```python
from build123d import *

# Parameters (mm, degrees)
F1_DEPTH = 40
F3_DEPTH = 12.5
F4_R     = 2.2
F5_DEPTH = 12.501
F7_SIZE  = 2
F6_R     = 4.65
F8_DEPTH = 1
F9_SIZE  = 2.44999


# Not quite as in the source:
# - a fillet or chamfer is up to 0.001 mm smaller than in the source, because OpenCascade refuses the exact size


with BuildPart() as f1:
    # F0 (on Top) → F1 (new body)
    with BuildSketch(Plane.XY):
        Polygon((2, 10), (-10.5, 10), (-10.5, 0), (0, 0), (0, -7.5), (1, -7.5), (5.5, -1), (2, -1), align=None)
    extrude(amount=F1_DEPTH)

    # F2 (on face) → F3 (cut, symmetric)
    with BuildSketch(Plane.XZ):
        with BuildLine():
            ThreePointArc((-2, 35.8), (-1, 34.8), (0, 35.8))
            Line((0, 35.8), (5.5, 35.8))
            Line((5.5, 35.8), (5.5, 40))
            Line((5.5, 40), (-10.5, 40))
            Line((-10.5, 40), (-10.5, 33.8))
            Line((-10.5, 33.8), (-3, 35.8))
            Line((-3, 35.8), (-2, 35.8))
        make_face()
    extrude(amount=F3_DEPTH, both=True, mode=Mode.SUBTRACT)

    # F4 (on face) → F5 (cut, through all)
    with BuildSketch(Plane.YZ.offset(2)):
        with Locations((4.5, 25.8)):
            Circle(F4_R)
        with Locations((4.5, 10)):
            Circle(F4_R)
    extrude(amount=-F5_DEPTH, mode=Mode.SUBTRACT)

    # F7
    f7_edges = [f1.edges().sort_by_distance(p)[0] for p in [
        (-10.5, 10, 16.9),
    ]]
    chamfer(f7_edges, length=F7_SIZE)

    # F6 (on face) → F8 (cut)
    with BuildSketch(Plane.YZ.offset(2)):
        with Locations((4.5, 25.8)):
            Circle(F6_R)
        with Locations((4.5, 10)):
            Circle(F6_R)
    extrude(amount=-F8_DEPTH, mode=Mode.SUBTRACT)

    # F9 (size 2.45 in the source; OpenCascade refuses exactly that, so slightly less here)
    f9_edges = [f1.edges().sort_by_distance(p)[0] for p in [
        (1, 2.3, 25.8),
        (1, 2.3, 10),
    ]]
    chamfer(f9_edges, length=F9_SIZE)


solid = f1.part
```
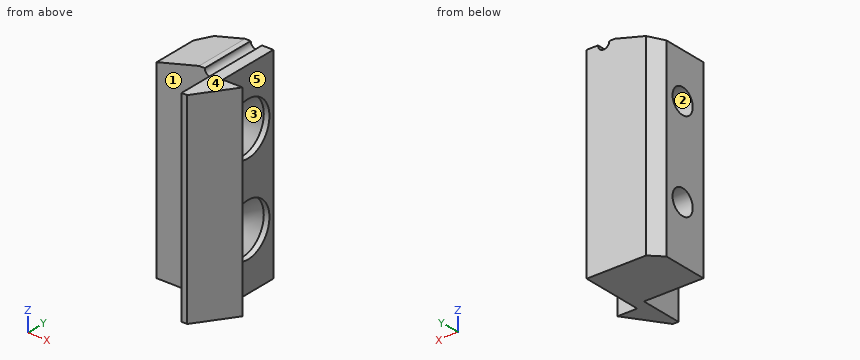
Read the model definition and answer for the solid it produces. Units are mm, in the model's axes. Face numbers are marked on the shaded views. A direction names the side the tool comes from. Coordinates: 2 decimals unless noted, no trailing zeros. Order: outer loops, then holes, each group sorted by start corner. A loop starts at its lowest first (then second) coordinate and runs counter-clockwise, first axis right, second up. Notation, with made-up numbers: (25.5, -27) - (71.5, -27) arc R26 ccw to (71.5, 5) - close; hole circle Ø8 at (30, 61.25). An arc over 180 degrees is marked (long way). Answer as a JSON object with one key per item and string values. Group by question number.
Item 1: Section D-D (z = 31.5) is taken. Give the vertices of the cut face in (x, y), plus the area to 3 significant figures.
Item 2: The mould has two halves that part along Z. Classify the marked faces 3, 4 and 5: +Z half, -Z half, draft (parallel to the pull), parting line (faces both ways), or undercut.
Item 3: Consider probe 1 along Z at (x, y) = (1.3, 4.5); probe 2 along Z at (x, y) = (-3.75, 4.5); probe 3 along X at (y, z) = (2.25, 20). Determine where each line is inside the solid, lowest interval first. Write a range as from..to.
Item 4: Section B-B (y = 4.5) is taken. State how many separate pieces and enclosed holes the cut face has, plus the area to 3 significant figures.
Item 5: Section C-C (x = -6) is taken. Give the vertices of the cut face in (y, z).
Item 6: A tool of negligible diameter and unlimited length cuts with its end or side. For the marked faces 1 and 2, from which of +Z, -Z, +X, -X, +Y, -Y can it reach the whole face along a straight path? Write none if from no direction.
Item 7: Flat-ended cylindrical pins translate along their axes: P1, Ø5, axis at x = -4.5, z = 17.5, coming from the -Y side; P2, Ø1, axis at x = 4.5, z = 17, coming from the +Y side; P3, Ø6, axis at y = 3.5, z = 27.5, coming from the +X side. Find the tip coordinate at first contact, or state that the pin passes through.
Results are:
{
 "1": {"outline": "(-10.5, 0) - (0, 0) - (0, -7.5) - (1, -7.5) - (5.5, -1) - (2, -1) - (2, 10) - (-8.5, 10) - (-10.5, 8) - close", "area": "146 mm^2"},
 "2": {"face 3": "undercut", "face 4": "+Z half", "face 5": "draft"},
 "3": {"probe 1": "z = 0..5.35, 14.65..21.15, 30.45..35.8", "probe 2": "z = 0..7.8, 12.2..23.6, 28..35.6", "probe 3": "x = -10.5..2"},
 "4": {"separate pieces": "3", "enclosed holes": "0", "area": "307 mm^2"},
 "5": {"outline": "(0, 0) - (10, 0) - (10, 35) - (0, 35) - close; hole circle Ø4.4 at (4.5, 10); hole circle Ø4.4 at (4.5, 25.8)"},
 "6": {"face 1": "+Z, -Z, -X, -Y", "face 2": "+X, -X"},
 "7": {"P1": "stops at y = 0", "P2": "stops at y = -1", "P3": "stops at x = 2"}
}
